```python
from build123d import *

# Parameters (mm, degrees)
SKETCH_1_R      = 2
SKETCH_1_R_2    = 1
EXTRUDE_1_DEPTH = 92
SKETCH_2_W      = 0.5
SKETCH_2_H      = 3
SKETCH_3_W      = 0.5
SKETCH_3_H      = 67


with BuildPart() as part:
    # Эскиз1 → Бобышка-Вытянуть1 (new body)
    with BuildSketch(Plane(origin=(0, 0, 0), x_dir=(1, 0, 0), z_dir=(0, 1, 0))):
        Circle(SKETCH_1_R)
        Circle(SKETCH_1_R_2, mode=Mode.SUBTRACT)
    extrude(amount=EXTRUDE_1_DEPTH)

    # Эскиз2 → Вырез-Повернуть1 (revolve, cut)
    with BuildSketch(Plane.XY):
        with Locations((1.75, 90.5)):
            Rectangle(SKETCH_2_W, SKETCH_2_H)
        with Locations((1.75, 83.5)):
            Rectangle(SKETCH_2_W, SKETCH_2_H)
    revolve(axis=Axis((0, 92, 0), (0, -1, 0)), mode=Mode.SUBTRACT)

    # Эскиз3 → Вырез-Повернуть2 (revolve, cut)
    with BuildSketch(Plane.XY):
        with Locations((1.75, 33.5)):
            Rectangle(SKETCH_3_W, SKETCH_3_H)
    revolve(axis=Axis((0, 0, 0), (0, 1, 0)), mode=Mode.SUBTRACT)


solid = part.part
```
Could you check a few things on this model? Use its own coordinates, in mm. A direction names the side the tool comes from. Coordinates: 2 decimals unless noted, no trailing zeros. Order: outer loops, then holes, each group sorted by start corner. A loop starts at its lowest first (then second) coordinate and runs counter-clockwise, first axis right, second up. Notation, with made-up numbers: M 20,2 L 48,2 A17 cw 48,7 Z; hole C 23,14.5 d5. An arc over 180 degrees is marked long. Use one line per item in the form item = value. Start each with the question number.
1. Please list where these lines run through material, in increasing order: line 1 (Y direction, x = 1.7, z = -0.75); line 2 (X direction, y = 27, z = 0); line 3 (Z direction, x = -0.1, y = 38).
2. Suppose I cut it at B-B on x = 0. Write out the boundary of the cut face in (y, z).
3. We'd pull the mould along X, two halves only. Please class faces 4 (the cylindrical face through (0, 45, 1)), 5 (the cylindrical face through (-1.5, 83.52, 0.07)): +X half, -X half, draft (parallel to the pull), parting line (faces both ways), or undercut.
4. Suppose I cut it at C-C on y = 28.5. Write out the boundary of the cut face in (x, z), then the cut area to 3 significant figures.
5. Suppose I cut it at A-A on z = 0. Write out the boundary of the cut face in (x, y), then the cut area to 3 significant figures.
6. On a 3-axis mill with a long thin cutter (end or side, diameter ignored), from which of +Z, -Z, +X, -X, +Y, -Y can I reach the whole of each face in a straight line? I mean faces 1 (the cylindrical face through (-1.5, 33.97, -0.07)), 2 (the cylindrical face through (0, 87, 2)), 3 (the cylindrical face through (-1.5, 90.52, 0.07)). Say none if no direction works.
Geometry says:
q1.line_1 = 67 to 82, 85 to 89
q1.line_2 = -1.5 to -1, 1 to 1.5
q1.line_3 = -1.5 to -0.99, 0.99 to 1.5
q2.outline = M 0,-1.5 L 67,-1.5 L 67,-2 L 82,-2 L 82,-1.5 L 85,-1.5 L 85,-2 L 89,-2 L 89,-1.5 L 92,-1.5 L 92,-1 L 0,-1 Z; M 0,1 L 92,1 L 92,1.5 L 89,1.5 L 89,2 L 85,2 L 85,1.5 L 82,1.5 L 82,2 L 67,2 L 67,1.5 L 0,1.5 Z
q3.face_4 = undercut
q3.face_5 = parting line
q4.outline = C 0,0 d3; hole C 0,0 d2
q4.area = 3.93 mm^2
q5.outline = M -2,67 L -1.5,67 L -1.5,0 L -1,0 L -1,92 L -1.5,92 L -1.5,89 L -2,89 L -2,85 L -1.5,85 L -1.5,82 L -2,82 Z; M 1,0 L 1.5,0 L 1.5,67 L 2,67 L 2,82 L 1.5,82 L 1.5,85 L 2,85 L 2,89 L 1.5,89 L 1.5,92 L 1,92 Z
q5.area = 111 mm^2
q6.face_1 = -Y
q6.face_2 = +Y, -Y
q6.face_3 = +Y
